Print and shaded views of the part. All mm, measured from the part's lowest x, y and z. A direction names the side the tool comes from. Give positions to 0.01 mm unless a question says otherwise; leave off trailing zeros. Write each loop counter-clockwise with the first axis right and the second up, starting at its lowest first coordinate (ties: lowest second). Pieces come first, ordered by that corner, then holes. Notation, with made-up numbers: (82.25, -8) -> (86.25, -8) arc R16 ccw to (86.25, -2) -> close; hole circle Ø6 at (40.5, 37). An arc over 180 degrees is marked (long way). Put each result on its own line as item: value.
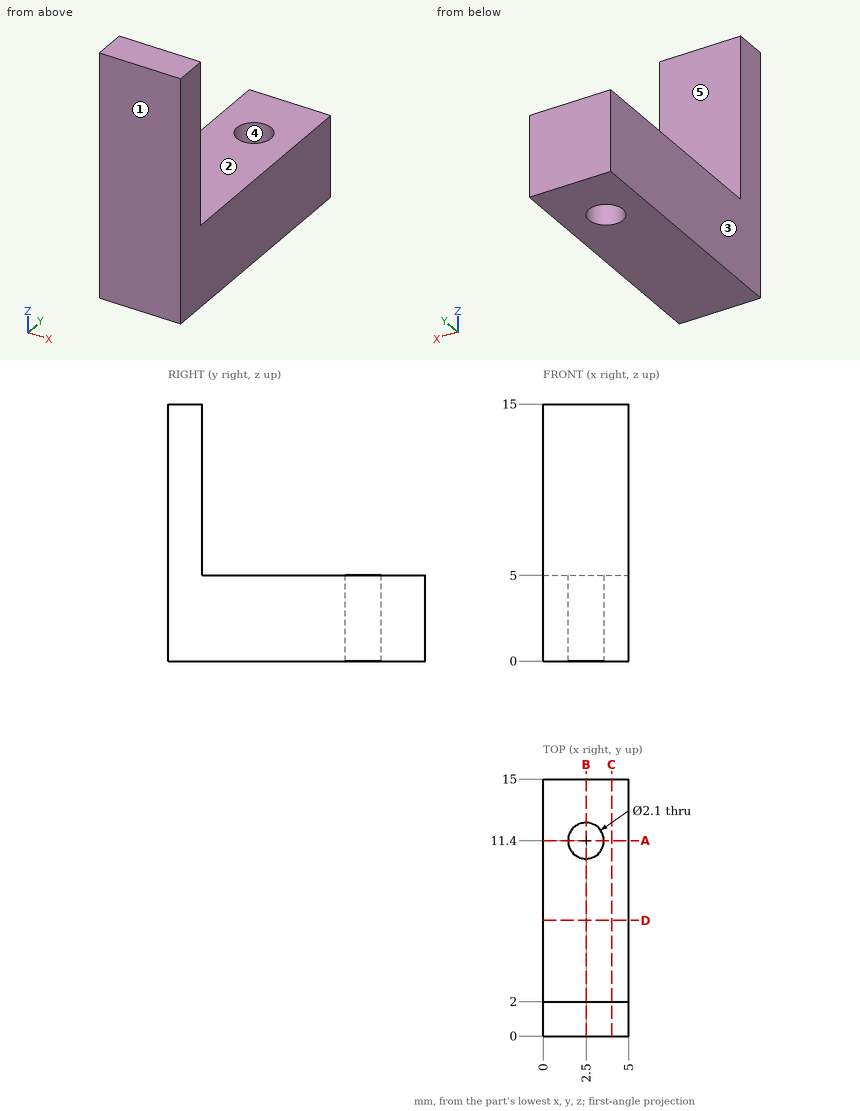
1) Slice it at D-D (y = 6.75). Write the cut outline in (x, z).
Filled sheet:
outline: (0, 0) -> (5, 0) -> (5, 5) -> (0, 5) -> close
2) Tool access for the marked faces 1 and 2: list every direction of +Z, -Z, +X, -X, +Y, -Y with a clear straight run to the whole face (end or side of a thin tool).
Filled sheet:
face 1: +Z, -Z, +X, -X, -Y
face 2: +Z, +X, -X, +Y
3) Slice it at C-C (x = 4). Write the cut outline in (y, z).
Filled sheet:
outline: (0, 0) -> (15, 0) -> (15, 5) -> (2, 5) -> (2, 15) -> (0, 15) -> close
4) Pull direction Y, two halves, no side cores. Call the marked faces 3, 4 and 5: released by +Y, released by -Y, zero draft, split by the parting line, or undercut.
Filled sheet:
face 3: zero draft
face 4: undercut
face 5: released by +Y
5) Wall check: L1, parallel to Y at x = 2.5, z = 2.85; L2, parallel to Y at x = 3.7, z = 10.5; L3, parallel to X at y = 11, z = 3.5. Give the ranges that are in metal, low to high.
Filled sheet:
L1: 0 to 10.35, 12.45 to 15
L2: 0 to 2
L3: 0 to 1.53, 3.47 to 5
6) Slice it at A-A (y = 11.4). Write the cut outline in (x, z).
Filled sheet:
outline: (0, 0) -> (1.45, 0) -> (1.45, 5) -> (0, 5) -> close; (3.55, 0) -> (5, 0) -> (5, 5) -> (3.55, 5) -> close
7) Slice it at B-B (x = 2.5). Write the cut outline in (y, z), plus the area to 3 significant figures.
Filled sheet:
outline: (0, 0) -> (10.35, 0) -> (10.35, 5) -> (2, 5) -> (2, 15) -> (0, 15) -> close; (12.45, 0) -> (15, 0) -> (15, 5) -> (12.45, 5) -> close
area: 84.5 mm2
8) Pin check, flat tip, straight feed: pin 1 (1 mm diameter, centred on x = 3.5, y = 5.5, fed in from +Z). Stop position of the tip, or through.
Filled sheet:
pin 1: z = 5
